from build123d import *

# Parameters (mm, degrees)
SKETCH12_R          = 80
BOSS_EXTRUDE1_DEPTH = 50
SKETCH13_R          = 25
CUT_EXTRUDE2_DEPTH  = 30
FILLET1_R           = 10
FILLET3_R           = 10
FILLET4_R           = 10


with BuildPart() as part:
    # Sketch12 → Boss-Extrude1 (new body)
    with BuildSketch(Plane(origin=(0, 0, 0), x_dir=(1, 0, 0), z_dir=(0, 1, 0))):
        with Locations(Location((80, 0, 0), (0, 0, 270))):
            Circle(SKETCH12_R)
    extrude(amount=BOSS_EXTRUDE1_DEPTH)

    # Sketch13 → Cut-Extrude2 (cut)
    with BuildSketch(Plane.XZ):
        with Locations(Location((80, 0, 0), (0, 0, 270))):
            Circle(SKETCH13_R)
    extrude(amount=-CUT_EXTRUDE2_DEPTH, mode=Mode.SUBTRACT)

    # Sketch14 → Cut-Revolve1 (revolve, cut)
    with BuildSketch(Plane.XY, mode=Mode.PRIVATE) as cut_revolve1_sk:
        Polygon((-7.132081461, 6.511492019), (0, 6.511492019), (13.618566057, 29.316874818), (13.618566057, 49.723955856), (-7.132081461, 49.723955856), align=None)
    revolve(cut_revolve1_sk.sketch.rotate(Axis((80, 0, 0), (0, 1, 0)), 270), axis=Axis((80, 0, 0), (0, 1, 0)), mode=Mode.SUBTRACT)

    # Fillet1
    fillet1_edges = [part.edges().sort_by_distance(p)[0] for p in [
        (80, 49.723955856, 66.381433943),
    ]]
    fillet(fillet1_edges, radius=FILLET1_R)

    # Fillet3
    fillet3_edges = [part.edges().sort_by_distance(p)[0] for p in [
        (160, 6.511492019, 0),
    ]]
    fillet(fillet3_edges, radius=FILLET3_R)

    # Fillet4
    fillet4_edges = [part.edges().sort_by_distance(p)[0] for p in [
        (80, 29.316874818, 66.381433943),
    ]]
    fillet(fillet4_edges, radius=FILLET4_R)


solid = part.part
Read the model definition and answer for the solid it produces. Units are mm, in the model's axes. A direction names the side the tool comes from. Coordinates: 2 decimals unless noted, no trailing zeros. Loops run counter-clockwise (first coordinate to the right, second up) from the corner with the lowest first, then second, coordinate; pieces in that order, holes last. Notation, with made-up numbers: (-2.5, 85.5) -> (7.5, 85.5) arc R8 ccw to (7.5, 98.5) -> close; hole circle Ø1 at (18.5, -3). An arc over 180 degrees is marked (long way). Write item = value, one per line. Start each with the question number.
1) For faces 5 (the face through (105.42, 35.95, -61.32)), 6 (the face through (99, 0, 17)), determine the directions among +Z, -Z, +X, -X, +Y, -Y from which every point of the face is accessible in a straight line to the end or side of a thin tool.
2) Find the intervals of material crossed by L1, parallel to X at y = 26, z = 19; L2, parallel to X at y = 11, z = 22.5; L3, parallel to Y at x = 107.5, z = 70.5, in increasing order. Write a range as from..to.
3) Given P1, Ø3, axis at x = 28.5, y = 23.5, coming from the -Z side; P2, Ø10, axis at x = 67.5, z = 63.5, coming from the -Y side; P3, Ø3, axis at y = 41, z = 37.5, coming from the -X side; P4, Ø2, axis at x = 134, z = 62, coming from the -Y side, each flat-ended and moving along its own axis, determine where each tip first touches the part or whether it passes through.
4) The mould has two halves that part along Z. Classify faces 1 (the face through (1.9, 1.85, -17.34)), 2 (the face through (55.594, 14.79, 5.42)), 3 (the face through (81, 50, -1)), 4 (the face through (80, 30, 0)): pulls with the +Z half, pulls with the -Z half, needs draft (parallel to the pull), parting line crosses it, or undercut.
5) The part is cut by section A-A, the plane y = 12. Determine the outline of the cut face in (x, z), plus the area to 3 significant figures.
Result:
q1.face_5 = none
q1.face_6 = +Z, -Z, +X, -X, -Y
q2.L1 = 14.33..63.75, 96.25..145.67
q2.L2 = 6.03..69.1, 90.9..153.97
q2.L3 = 0..13.76, 49.7..50
q3.P1 = -49.25
q3.P2 = 0
q3.P3 = 24.09
q3.P4 = through
q4.face_1 = parting line crosses it
q4.face_2 = undercut
q4.face_3 = needs draft
q4.face_4 = undercut
q5.outline = circle Ø153.44 at (80, 0); hole circle Ø50 at (80, 0)
q5.area = 16,500 mm²
